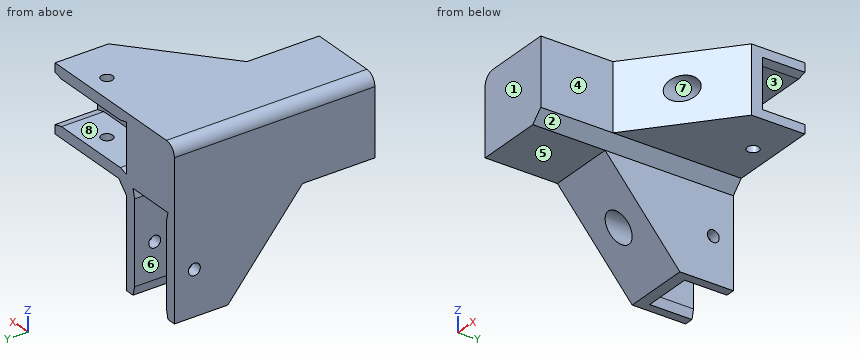
```python
from build123d import *

# Parameters (mm, degrees)
SKETCH1_W                = 75
SKETCH1_H                = 75
BOSS_EXTRUDE1_DEPTH      = 90
SKETCH2_W                = 45
SKETCH2_H                = 20
SKETCH2_W_2              = 20
SKETCH2_H_2              = 45
CUT_EXTRUDE2_DEPTH       = 19
SKETCH3_W                = 45
SKETCH3_H                = 45
CUT_EXTRUDE3_DEPTH       = 140.104277432
CUT_EXTRUDE4_DEPTH       = 140.104277432
CUT_EXTRUDE5_DEPTH       = 126.49900398
FILLET1_R                = 5
CUT_EXTRUDE10_DEPTH      = 126.49900398
CUT_EXTRUDE10_DEPTH_BACK = 126.49900398
SKETCH7_R                = 2.65
CUT_EXTRUDE11_DEPTH      = 126.49900398
CUT_EXTRUDE11_DEPTH_BACK = 126.49900398
SKETCH8_R                = 2.65
SKETCH9_R                = 2.65
CUT_EXTRUDE12_DEPTH      = 128.636201761
SKETCH10_R               = 5.5
CUT_EXTRUDE13_DEPTH      = 125.923976882
CHAMFER3_SIZE            = 5
CUT_EXTRUDE14_DEPTH      = 19


with BuildPart() as part:
    # Sketch1 → Boss-Extrude1 (new body)
    with BuildSketch(Plane(origin=(0, 0, 0), x_dir=(1, 0, 0), z_dir=(0, 1, 0))):
        with Locations((37.5, 37.5)):
            Rectangle(SKETCH1_W, SKETCH1_H)
    extrude(amount=BOSS_EXTRUDE1_DEPTH)

    # Sketch2 → Cut-Extrude2 (cut)
    with BuildSketch(Plane(origin=(0, 90, 0), x_dir=(1, 0, 0), z_dir=(0, 1, 0))):
        with Locations((52.5, 15)):
            Rectangle(SKETCH2_W, SKETCH2_H)
        with Locations((15, 52.5)):
            Rectangle(SKETCH2_W_2, SKETCH2_H_2)
    extrude(amount=-CUT_EXTRUDE2_DEPTH, mode=Mode.SUBTRACT)

    # Sketch3 → Cut-Extrude3 (cut, through all)
    with BuildSketch(Plane(origin=(0, 90, 0), x_dir=(1, 0, 0), z_dir=(0, 1, 0))):
        with Locations((52.5, 52.5)):
            Rectangle(SKETCH3_W, SKETCH3_H)
    extrude(amount=-CUT_EXTRUDE3_DEPTH, mode=Mode.SUBTRACT)

    # Sketch4 → Cut-Extrude4 (cut, through all)
    with BuildSketch(Plane.XY):
        Polygon((35, 32.436014753), (35, 0), (75, 0), (75, 66), align=None)
    extrude(amount=-CUT_EXTRUDE4_DEPTH, mode=Mode.SUBTRACT)

    # Sketch5 → Cut-Extrude5 (cut, through all)
    with BuildSketch(Plane(origin=(30, 0, 0), x_dir=(0, 0, -1), z_dir=(1, 0, 0))):
        Polygon((35, 0), (35, 32.436014753), (75, 66), (75, 0), align=None)
    extrude(amount=-CUT_EXTRUDE5_DEPTH, mode=Mode.SUBTRACT)

    # Fillet1
    fillet1_edges = [part.edges().sort_by_distance(p)[0] for p in [
        (0, 45, 0),
    ]]
    fillet(fillet1_edges, radius=FILLET1_R)

    # Sketch7 → Cut-Extrude10 (cut, two sides: drawn at the far end of the back side and taken through both)
    with BuildSketch(Plane(origin=(0, 0, -30), x_dir=(-1, 0, 0), z_dir=(0, 0, -1)).offset(-CUT_EXTRUDE10_DEPTH_BACK)):
        with Locations((-55, 81)):
            Circle(SKETCH7_R)
    extrude(amount=CUT_EXTRUDE10_DEPTH + CUT_EXTRUDE10_DEPTH_BACK, mode=Mode.SUBTRACT)

    # Sketch8 → Cut-Extrude11 (cut, two sides: drawn at the far end of the back side and taken through both)
    with BuildSketch(Plane(origin=(30, 0, 0), x_dir=(0, 0, -1), z_dir=(1, 0, 0)).offset(-CUT_EXTRUDE11_DEPTH_BACK)):
        with Locations((55, 81)):
            Circle(SKETCH8_R)
    extrude(amount=CUT_EXTRUDE11_DEPTH + CUT_EXTRUDE11_DEPTH_BACK, mode=Mode.SUBTRACT)

    # Sketch9 → Cut-Extrude12 (cut, through all)
    with BuildSketch(Plane(origin=(0, 71, 0), x_dir=(1, 0, 0), z_dir=(0, 1, 0))):
        with Locations(Location((15, 55, 0), (0, 0, 270))):
            Circle(SKETCH9_R)
        with Locations(Location((55, 15, 0), (0, 0, 270))):
            Circle(SKETCH9_R)
    extrude(amount=-CUT_EXTRUDE12_DEPTH, mode=Mode.SUBTRACT)

    # Sketch10 → Cut-Extrude13 (cut, through all)
    with BuildSketch(Plane(origin=(0, 66, 0), x_dir=(1, 0, 0), z_dir=(0, 1, 0))):
        with Locations(Location((55, 15, 0), (0, 0, 270))):
            Circle(SKETCH10_R)
        with Locations(Location((15, 55, 0), (0, 0, 270))):
            Circle(SKETCH10_R)
    extrude(amount=-CUT_EXTRUDE13_DEPTH, mode=Mode.SUBTRACT)

    # Chamfer3
    chamfer3_edges = [part.edges().sort_by_distance(p)[0] for p in [
        (30, 45, -30),
    ]]
    chamfer(chamfer3_edges, length=CHAMFER3_SIZE - 0.0001)  # a hair under: the kernel refuses the full size

    # Sketch11 → Cut-Extrude14 (cut)
    with BuildSketch(Plane(origin=(0, 90, 0), x_dir=(1, 0, 0), z_dir=(0, 1, 0))):
        Polygon((5, 30), (4, 30), (5, 34), align=None)
        Polygon((25, 30), (26, 30), (25, 34), align=None)
        Polygon((30, 25), (34, 25), (30, 26), align=None)
        Polygon((30, 5), (30, 4), (34, 5), align=None)
        Polygon((25, 75), (26, 75), (25, 71), align=None)
        Polygon((5, 71), (5, 75), (4, 75), align=None)
        Polygon((75, 5), (71, 5), (75, 4), align=None)
        Polygon((71, 25), (75, 25), (75, 26), align=None)
    extrude(amount=-CUT_EXTRUDE14_DEPTH, mode=Mode.SUBTRACT)


solid = part.part
```
Verification items for the finished model (mm, model axes). Face numbers are marked on the shaded views. A direction names the side the tool comes from. Coordinates: 2 decimals unless noted, no trailing zeros. Loops run counter-clockwise (first coordinate to the right, second up) from the corner with the lowest first, then second, coordinate; pieces in that order, holes last. Notation, with made-up numbers: (0.5, 83.25) -> (40.5, 83.25) arc R11 ccw to (40.5, 98.25) -> close; hole circle Ø6 at (-38.75, 13). An arc over 180 degrees is marked (long way). Answer in a Markdown table with one row per item. Add a question column.
1. Draft check along Z on the marked faces 1, 2 and 3. Enter one of: +Z half, -Z half, draft (parallel to the pull), parting line (faces both ways), or undercut.
2. Depth check by flat-ended pin: P1, Ø9, axis at x = 15, z = -55, coming from the +Y side; P2, Ø2, axis at y = 68, z = -46, coming from the +X side; P3, Ø9, axis at x = 54.5, z = -17, coming from the -Y side; P4, Ø5, axis at x = 55, y = 81, coming from the -Z side. Enter the tip coordinate at first touch or a pass-through.
3. Section check A-A, the plane z = -56. Enter the section's corners in (x, y), then the cut area to 3 significant figures.
4. Section check C-C, the plane x = 15. Enter the section's corners in (y, z), then the cut area to 3 significant figures.
5. Material ranges on probe 1 along X at (y, z) = (86, -59); probe 2 along X at (y, z) = (67, -55); probe 3 along Z at (x, y) = (46, 84), recorded low to high. Write a range as [from, to].
6. Access from +Z, -Z, +X, -X, +Y, -Y to the whole of each face (thin tool, end or side, straight path). Record for the marked faces 4, 5, 6, 7 and 8.
7. Section check D-D, the plane z = -15. Enter the section's corners in (x, y), then the cut area to 3 significant figures.
Derived:
| question | item | result |
|---|---|---|
| 1 | face 1 | draft |
| 1 | face 2 | -Z half |
| 1 | face 3 | undercut |
| 2 | P1 | stops at y = 71 |
| 2 | P2 | stops at x = 30 |
| 2 | P3 | stops at y = 45.03 |
| 2 | P4 | passes through |
| 3 | outline | (0, 50.06) -> (9.59, 50.06) -> (9.59, 66) -> (12.55, 66) -> (12.55, 71) -> (5, 71) -> (5, 78.55) -> (0, 78.55) -> close; (0, 83.45) -> (5, 83.45) -> (5, 90) -> (0, 90) -> close; (17.45, 66) -> (20.41, 66) -> (20.41, 50.06) -> (30, 50.06) -> (30, 78.55) -> (25, 78.55) -> (25, 71) -> (17.45, 71) -> close; (25, 83.45) -> (30, 83.45) -> (30, 90) -> (25, 90) -> close |
| 3 | area | 572 mm² |
| 4 | outline | (0, -35) -> (32.44, -35) -> (44.6, -49.5) -> (66, -49.5) -> (66, -52.35) -> (71, -52.35) -> (71, -30) -> (90, -30) -> (90, 0) -> (0, 0) -> close; (53.83, -60.5) -> (66, -75) -> (71, -75) -> (71, -57.65) -> (66, -57.65) -> (66, -60.5) -> close |
| 4 | area | 3,720 mm² |
| 5 | probe 1 | x = [0, 5], [25, 30] |
| 5 | probe 2 | x = [0, 12.35], [17.65, 30] |
| 5 | probe 3 | z = [-30, -25], [-5, 0] |
| 6 | face 4 | +Z, -Z, +X, -Y |
| 6 | face 5 | -Z, +X, -X, -Y |
| 6 | face 6 | -Z, +Y |
| 6 | face 7 | -Y |
| 6 | face 8 | +X, +Y |
| 7 | outline | (0, 0) -> (35, 0) -> (35, 32.44) -> (49.5, 44.6) -> (49.5, 66) -> (52.35, 66) -> (52.35, 71) -> (30, 71) -> (30, 90) -> (0, 90) -> close; (57.65, 66) -> (60.5, 66) -> (60.5, 53.83) -> (75, 66) -> (75, 71) -> (57.65, 71) -> close |
| 7 | area | 3,720 mm² |
